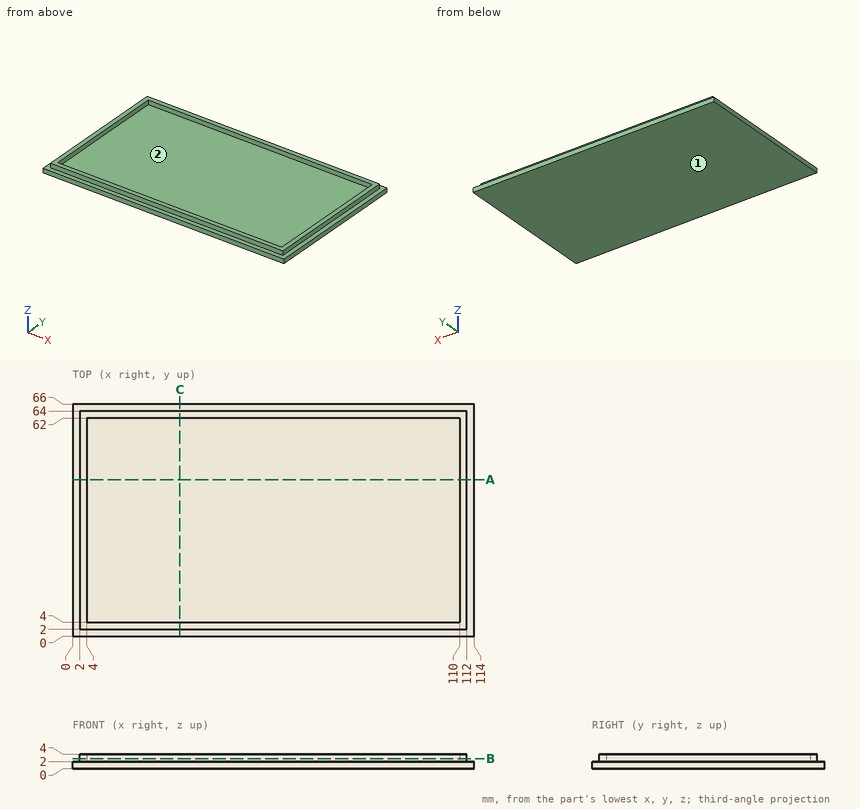
Check sheet for the drawn part. Datum: minimum x, y, z corner. Units: mm. Round coordinates to 2 decimals unless told otherwise and drop trailing zeros. Loops run counter-clockwise (first coordinate to the right, second up) from the corner with the lowest first, then second, coordinate; pieces in that order, holes last. Notation, with made-up numbers: (-21.5, 84.25) - (13.5, 84.25) arc R19 cw to (13.5, 89.25) - close; hole circle Ø8 at (51, 10.5). An arc over 180 degrees is marked (long way). Use one line per item in the form item = value.
1. Scan lines: probe 1 along X at (y, z) = (10, 3.55); probe 2 along Y at (x, z) = (9.5, 2.2); probe 3 along Z at (x, y) = (39, 21.5). Record each from-to range of solid material in increasing order.
A:
probe_1 = 2 to 4, 110 to 112
probe_2 = 2 to 4, 62 to 64
probe_3 = 0 to 2
2. Section check C-C on x = 30.5. Record the cut outline in (y, z).
A:
outline = (0, 0) - (66, 0) - (66, 2) - (64, 2) - (64, 4) - (62, 4) - (62, 2) - (4, 2) - (4, 4) - (2, 4) - (2, 2) - (0, 2) - close
3. Gauge pin test, flat ends, axial feed: pin 1 Ø0.6 at (y, z) = (32.5, 3) entering from +X; pin 2 Ø1 at (x, z) = (72.5, 3) entering from +Y; pin 3 Ø2 at (y, z) = (46, 3.5) entering from -X. Record the tip position at first contact, or that the pin passes through.
A:
pin_1 = 112
pin_2 = 64
pin_3 = 2
4. Section check A-A on y = 44.5. Record the cut outline in (x, z).
A:
outline = (0, 0) - (114, 0) - (114, 2) - (112, 2) - (112, 4) - (110, 4) - (110, 2) - (4, 2) - (4, 4) - (2, 4) - (2, 2) - (0, 2) - close
5. Section check B-B on z = 2.8. Record the cut outline in (x, y), and give its area (3 significant figures).
A:
outline = (2, 2) - (112, 2) - (112, 64) - (2, 64) - close; hole (4, 4) - (110, 4) - (110, 62) - (4, 62) - close
area = 672 mm²
6. Draft check along Y on the marked faces 1 and 2. Enter one of: pulls with the +Y half, pulls with the -Y half, needs draft (parallel to the pull), parting line crosses it, or undercut.
A:
face_1 = needs draft
face_2 = undercut
